from build123d import *

# Parameters (mm, degrees)
CROQUIS1_W              = 600
CROQUIS1_H              = 600
CROQUIS1_R              = 187.5
SALIENTE_EXTRUIR1_DEPTH = 100
CORTAR_EXTRUIR6_DEPTH   = 80
CORTAR_EXTRUIR7_DEPTH   = 80
CORTAR_EXTRUIR8_DEPTH   = 80
CORTAR_EXTRUIR9_DEPTH   = 80


with BuildPart() as part:
    # Croquis1 → Saliente-Extruir1 (new body)
    with BuildSketch(Plane.XY):
        with Locations((24.047372846, 17.859468054)):
            Rectangle(CROQUIS1_W, CROQUIS1_H)
        with Locations((24.047372846, 17.859468054)):
            Circle(CROQUIS1_R, mode=Mode.SUBTRACT)
    extrude(amount=SALIENTE_EXTRUIR1_DEPTH)

    # Croquis2 → Cortar-Extruir6 (cut)
    with BuildSketch(Plane.ZY.offset(275.952627154)):
        Polygon((80, -192.140531946), (0, 227.859468054), (0, -192.140531946), align=None)
    extrude(amount=-CORTAR_EXTRUIR6_DEPTH, mode=Mode.SUBTRACT)

    # Croquis3 → Cortar-Extruir7 (cut)
    with BuildSketch(Plane.XZ.offset(282.140531946)):
        Polygon((234.047372846, 80), (-185.952627154, 0), (234.047372846, 0), align=None)
    extrude(amount=-CORTAR_EXTRUIR7_DEPTH, mode=Mode.SUBTRACT)

    # Croquis4 → Cortar-Extruir8 (cut)
    with BuildSketch(Plane(origin=(324.047372846, 0, 0), x_dir=(0, 0, -1), z_dir=(1, 0, 0))):
        Polygon((-80, 227.859468054), (0, -192.140531946), (0, 227.859468054), align=None)
    extrude(amount=-CORTAR_EXTRUIR8_DEPTH, mode=Mode.SUBTRACT)

    # Croquis6 → Cortar-Extruir9 (cut)
    with BuildSketch(Plane(origin=(0, 317.859468054, 0), x_dir=(1, 0, 0), z_dir=(0, 1, 0))):
        Polygon((234.047372846, 0), (-185.952627154, 0), (-185.952627154, -80), align=None)
    extrude(amount=-CORTAR_EXTRUIR9_DEPTH, mode=Mode.SUBTRACT)


solid = part.part
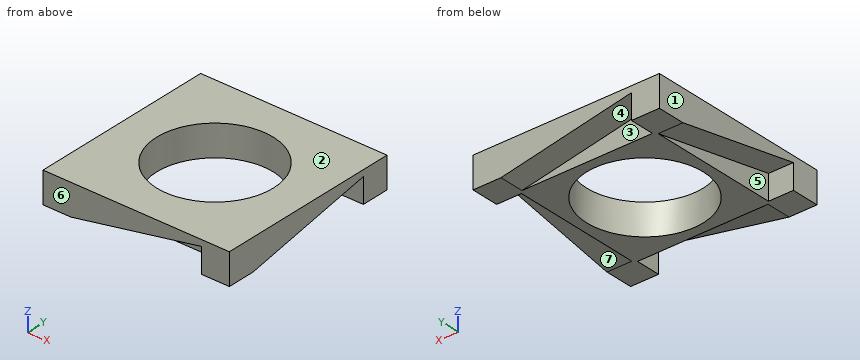
Input: part model. Units: mm. Frame: model coordinates. Face numbers are marked on the shaded views. A direction names the side the tool comes from. Round coordinates to 2 decimals unless told otherwise and drop trailing zeros. Loops run counter-clockwise (first coordinate to the right, second up) from the corner with the lowest first, then second, coordinate; pieces in that order, holes last. Notation, with made-up numbers: (30.25, -24) -> (75.25, -24) arc R14 cw to (75.25, -4) -> close; hole circle Ø3 at (75.5, -17.75). An arc over 180 degrees is marked (long way). Answer as a JSON object with one key per item and string values. Group by question number.
1) Section query B-B on x = -79. Output: boundary loops of the cut face in (y, z) (3 decimals).
2) Section query A-A on y = -24. Output: boundary loops of the cut face in (x, z), plus the area to 3 significant figures.
3) Section query C-C on z = 70. Output: boundary loops of the cut face in (x, y).
4) Draft query along X for the marked faces 1, 2 and 3. Return one class per face: +X half, -X half, draft (parallel to the pull), parting line (faces both ways), or undercut.
5) Section query D-D on x = 286.5. Output: boundary loops of the cut face in (y, z).
6) Reachability of the marked faces 4, 5, 6 and 7 from +Z, -Z, +X, -X, +Y, -Y: full face, straight path, thin tool, end or side. Return the list, or none.
7) Ray query, L1, parallel to Y at x = -170.5, z = 75.5; L2, parallel to X at y = -145, z = 6; L3, parallel to Y at x = -63, z = 40. Return the intervals inside material, ascending.
8) Pin query (flat end, axial travel): pin 1 (2 mm diameter, centred on y = 205.5, z = 37.5, fed in from +X); pin 2 (6 mm diameter, centred on y = 68, z = 24, fed in from -X); pin 3 (8 mm diameter, centred on x = 96, z = 22, fed in from +Y). Return the tip coordinate at first contact, or that it passes through.
Reply:
{
 "1": {"outline": "(-282.141, 20.372) -> (-202.141, 20.372) -> (-202.141, 0) -> (-138.785, 0) -> (-138.785, 100) -> (-282.141, 100) -> close; (174.504, 0) -> (237.859, 0) -> (237.859, 59.628) -> (317.859, 59.628) -> (317.859, 100) -> (174.504, 100) -> close"},
 "2": {"outline": "(-275.95, 47.97) -> (-195.95, 47.97) -> (-195.95, 0) -> (-158.72, 0) -> (-158.72, 100) -> (-275.95, 100) -> close; (206.82, 0) -> (244.05, 0) -> (244.05, 32.03) -> (324.05, 32.03) -> (324.05, 100) -> (206.82, 100) -> close", "area": "17,000 mm2"},
 "3": {"outline": "(-275.95, -282.14) -> (181.55, -282.14) -> (181.55, -202.14) -> (234.05, -202.14) -> (234.05, -282.14) -> (324.05, -282.14) -> (324.05, 175.36) -> (244.05, 175.36) -> (244.05, 227.86) -> (324.05, 227.86) -> (324.05, 317.86) -> (-133.45, 317.86) -> (-133.45, 237.86) -> (-185.95, 237.86) -> (-185.95, 317.86) -> (-275.95, 317.86) -> (-275.95, -139.64) -> (-195.95, -139.64) -> (-195.95, -192.14) -> (-275.95, -192.14) -> close; hole circle Ø375 at (24.05, 17.86)"},
 "4": {"face 1": "-X half", "face 2": "draft", "face 3": "undercut"},
 "5": {"outline": "(-282.14, 0) -> (-192.14, 0) -> (227.86, 80) -> (227.86, 0) -> (317.86, 0) -> (317.86, 100) -> (-282.14, 100) -> close"},
 "6": {"face 4": "-Z, +Y", "face 5": "-Z, -X", "face 6": "+Z, -Z, +X, -X, -Y", "face 7": "-Z, +X"},
 "7": {"L1": "y = -282.14 to 237.86", "L2": "x = -195.95 to -68.87, 116.96 to 244.05", "L3": "y = -282.14 to -148.21, 183.93 to 237.86"},
 "8": {"pin 1": "stops at x = 244.05", "pin 2": "stops at x = -195.95", "pin 3": "stops at y = 237.86"}
}
